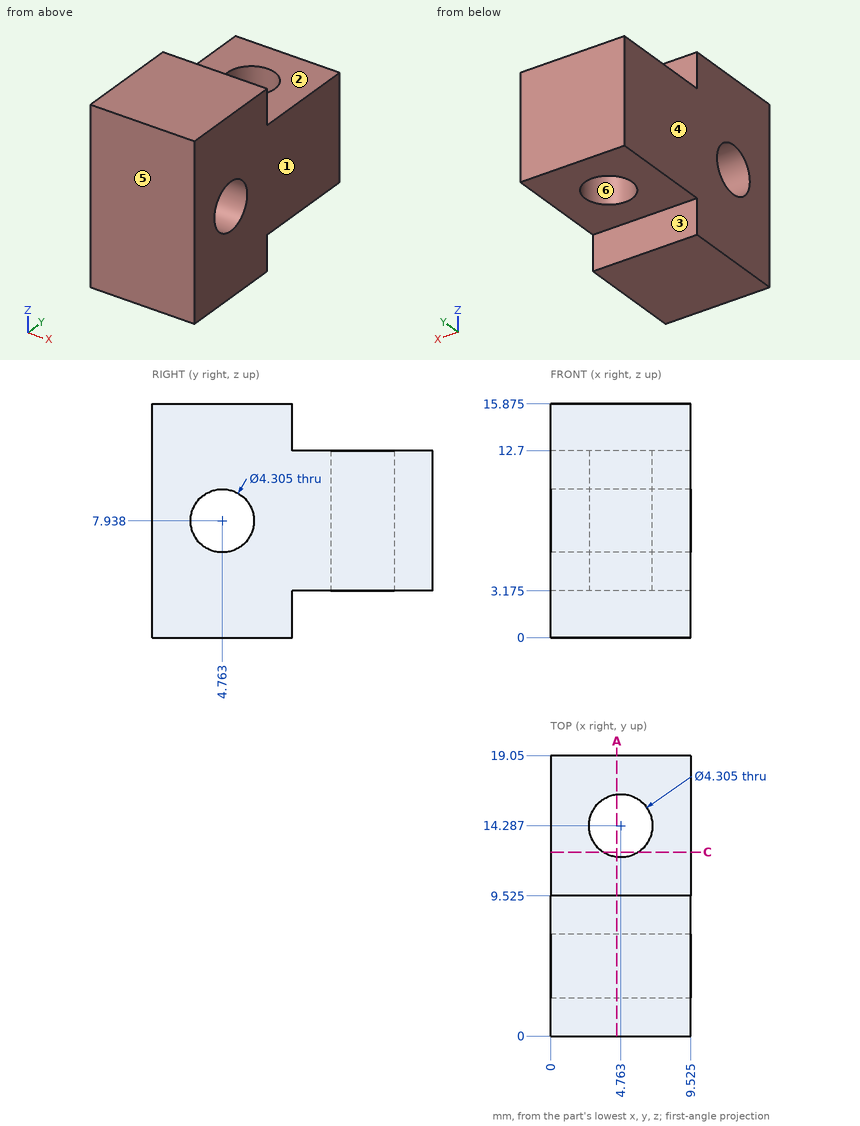
Geometry: see drawing. Coordinates: mm, zero at the bounding-box minimum. A direction names the side the tool comes from. Give positions to 0.01 mm unless a question says otherwise; leave off trailing zeros. Loops run counter-clockwise (first coordinate to the right, second up) from the corner with the lowest first, then second, coordinate; pieces in that order, holes last. Notation, with made-up numbers: (89.25, 51) - (145.25, 51) arc R18 cw to (145.25, 78) - close; hole circle Ø8 at (68, 3.25). An arc over 180 degrees is marked (long way). Use CSV: the item, a comma, the result in double quotes.
1) Mould query, pull axis X, two halves, no side actions, for the marked faces 4, 5 and 6. Classes: +X half, -X half, draft (parallel to the pull), parting line (faces both ways), or undercut.
Worked out:
face 4,"-X half"
face 5,"draft"
face 6,"undercut"
2) Cut plane A-A (x = 4.5). Count the separate pieces of the cut face and the enclosed holes in it, and give its area (3 significant figures).
Worked out:
separate pieces,"2"
enclosed holes,"1"
area,"187 mm^2"
3) Cut plane C-C (y = 12.5). Output: boundary loops of the cut face in (x, z) (1 decimal).
Worked out:
outline,"(0, 3.2) - (3.6, 3.2) - (3.6, 12.7) - (0, 12.7) - close; (6, 3.2) - (9.5, 3.2) - (9.5, 12.7) - (6, 12.7) - close"
4) Pin query (flat end, axial travel): P1, Ø3, axis at y = 7, z = 6, coming from the -X side; P2, Ø3, axis at x = 6.5, y = 13.5, coming from the -Z side (1 decimal); P3, Ø3, axis at x = 5, y = 12, coming from the +Z side; P4, Ø1.6, axis at x = 4, z = 1, coming from the +Y side (1 decimal). Return the tip coordinate at first contact, or that it passes through.
Worked out:
P1,"stops at x = 0"
P2,"stops at z = 3.2"
P3,"stops at z = 12.7"
P4,"stops at y = 9.5"
5) Line query: line 1 (Y direction, x = 2.75, z = 15) (1 decimal); line 2 (Y direction, x = 3.75, z = 7.25); line 3 (Z direction, x = 3, y = 18.25) (1 decimal). Output: solid intervals per line, ascending.
Worked out:
line 1,"y = 0 to 9.5"
line 2,"y = 0 to 2.72, 6.8 to 12.39, 16.19 to 19.05"
line 3,"z = 3.2 to 12.7"
6) Set-up query: the marked faces 1, 2 and 3. Return all of +Z, -Z, +X, -X, +Y, -Y with unobstructed straight access to the full face (end or side cutting, diameter ignored); none if empty.
Worked out:
face 1,"+Z, -Z, +X, +Y, -Y"
face 2,"+Z, +X, -X, +Y"
face 3,"-Z, +X, -X, +Y"
